Read the model definition and answer for the solid it produces. Units are mm, in the model's axes. Give positions to 0.01 mm unless a question says otherwise; leave off trailing zeros. Loops run counter-clockwise (first coordinate to the right, second up) from the corner with the lowest first, then second, coordinate; pieces in that order, holes last. Notation, with made-up numbers: (60, 59) - (81, 59) arc R28 cw to (81, 87) - close; hole circle Ø10 at (-38, 66.5). An arc over 180 degrees is marked (long way). Write item = value, one per line.
```python
from build123d import *

# Parameters (mm, degrees)
SKETCH1_R           = 4.75
BOSS_EXTRUDE1_DEPTH = 20
CHAMFER1_SIZE       = 1.5
CHAMFER2_SIZE       = 1.5
SCALE1_SCALE        = 0.75
SCALE2_SCALE        = 0.85


with BuildPart() as part:
    # Sketch1 → Boss-Extrude1 (new body)
    with BuildSketch(Plane(origin=(0, 0, 0), x_dir=(0, 1, 0), z_dir=(0, 0, 1))):
        Circle(SKETCH1_R)
    extrude(amount=BOSS_EXTRUDE1_DEPTH)

    # Chamfer1
    chamfer1_edges = [part.edges().sort_by_distance(p)[0] for p in [
        (0, -4.75, 0),
    ]]
    chamfer(chamfer1_edges, length=CHAMFER1_SIZE)

    # Chamfer2
    chamfer2_edges = [part.edges().sort_by_distance(p)[0] for p in [
        (0, -4.75, 20),
    ]]
    chamfer(chamfer2_edges, length=CHAMFER2_SIZE)


with BuildPart() as part_1:
    # Scale1: scaled about (0, 0, 10)
    add(part.part.scale(SCALE1_SCALE).moved(Location((0, 0, 2.5))))


with BuildPart() as part_2:
    # Scale2: scaled about (0, 0, 10)
    add(part_1.part.scale(SCALE2_SCALE).moved(Location((0, 0, 1.5))))


solid = part_2.part
```
1) A cutting plane is placed at A-A on x = 0. Determine the outline of the cut face in (y, z) (3 decimals), then the cut area to 3 significant figures.
Output:
outline = (-3.028, 4.581) - (-2.072, 3.625) - (2.072, 3.625) - (3.028, 4.581) - (3.028, 15.419) - (2.072, 16.375) - (-2.072, 16.375) - (-3.028, 15.419) - close
area = 75.4 mm²
2) A cutting plane is placed at C-C on z = 8.25. Determine the outline of the cut face in (x, y), then the cut area to 3 significant figures.
Output:
outline = circle Ø6.06 at (0, 0)
area = 28.8 mm²
3) Each of these flat-tipped pins is pushed along its axis until it touches: P1, Ø2, axis at x = 2.5, z = 11.5, coming from the +Y side; P2, Ø1, axis at x = -1, z = 5, coming from the -Y side. Where does it stop, or does it pass through?
Output:
P1 = 2.63
P2 = -2.99
4) Find the intervals of material crossed by probe 1 along Y at (x, z) = (1, 5.25); probe 2 along X at (y, z) = (-1.5, 6.25); probe 3 along Y at (x, z) = (-0.5, 13), in increasing order.
Output:
probe_1 = -2.86 to 2.86
probe_2 = -2.63 to 2.63
probe_3 = -2.99 to 2.99
